```python
from build123d import *

# Parameters (mm, degrees)
F0_R          = 12.5
F1_DEPTH      = 10
F2_DEPTH      = 15
F2_DEPTH_BACK = 5


with BuildPart() as f1:
    # F0 (on Top) → F1 (new body)
    with BuildSketch(Plane.XY):
        with BuildLine():
            ThreePointArc((14.990479, 0.534354), (14.99762, 0.267219), (15, 0))
            ThreePointArc((15, 0), (-1.712048, -14.901976), (-14.609185, 3.401721))
            Line((-14.609185, 3.401721), (-48, -140))
            Line((-48, -140), (-78, -140))
            Line((-78, -140), (-78, -150))
            Line((-78, -150), (50, -150))
            Line((50, -150), (50, -140))
            Line((50, -140), (20, -140))
            Line((20, -140), (14.990479, 0.534354))
        make_face()
        with BuildLine():
            ThreePointArc((-14.609185, 3.401721), (-1.712048, -14.901976), (15, 0))
            ThreePointArc((15, 0), (14.99762, 0.267219), (14.990479, 0.534354))
            ThreePointArc((14.990479, 0.534354), (1.446304, 14.930111), (-14.609185, 3.401721))
        make_face()
        Circle(F0_R, mode=Mode.SUBTRACT)
    extrude(amount=F1_DEPTH)

    # F0 (on Top) → F2 (join, two sides)
    with BuildSketch(Plane.XY) as f2_sk:
        with BuildLine():
            ThreePointArc((-14.609185, 3.401721), (-1.712048, -14.901976), (15, 0))
            ThreePointArc((15, 0), (14.99762, 0.267219), (14.990479, 0.534354))
            ThreePointArc((14.990479, 0.534354), (1.446304, 14.930111), (-14.609185, 3.401721))
        make_face()
        Circle(F0_R, mode=Mode.SUBTRACT)
    extrude(amount=F2_DEPTH)
    extrude(f2_sk.sketch, amount=-F2_DEPTH_BACK)


solid = f1.part
```
CAD build for the part. Positions are in the model's coordinates, mm. A direction names the side the tool comes from. Give positions to 0.01 mm unless a question says otherwise; leave off trailing zeros. Write each loop counter-clockwise with the first axis right and the second up, starting at its lowest first coordinate (ties: lowest second). Pieces come first, ordered by that corner, then holes. Notation, with made-up numbers: M 10,76.25 L 64,76.25 A23 cw 64,91.25 Z; hole C 13.25,-15.5 d5. An arc over 180 degrees is marked long. Return JSON: item names as keys, results as strings. Group by question number.
(1) 3-axis set-ups, long thin cutter, end or side, ignore diameter. For faces 1 (the face through (-63, -140, 5)), 2 (the face through (-3.4, 12.3, 15)), 3 (the face through (35, -140, 5)): which of +Z, -Z, +X, -X, +Y, -Y reach the whole face in a straight line?
(2) Drill centre lines: L1, parallel to Y at x = 0, z = -3.6; L2, parallel to Y at x = 0, z = 7; L3, parallel to Y at x = 39, z = 3.75. Where is each one in solid material? Low to high. Write a range as [from, to].
(3) Band-saw the part on D-D (y = -108). Give the cut face in (x, z), and give its area (3 significant figures).
(4) Band-saw the part on B-B (z = 7.25). Give the cut face in (x, y).
(5) Flat gauge pins, fed straight in: pin 1 Ø1 at (x, y) = (5.5, -70) entering from +Z; pin 2 Ø20 at (x, y) = (0, 0) entering from +Z; pin 3 Ø3 at (x, z) = (40, 4) entering from +Y; pin 4 Ø10 at (x, y) = (-29, -43) entering from -Z. Where does each tip first touch, or does it go through?
(6) Band-saw the part on C-C (z = -2). Give the cut face in (x, y).
(7) Band-saw the part on A-A (x = 0). Give the cut face in (y, z).
Entries:
{
 "1": {"face 1": "+Z, -Z, -X, +Y", "face 2": "+Z, +X, -X, +Y, -Y", "face 3": "+Z, -Z, +X, +Y"},
 "2": {"L1": "y = [-15, -12.5], [12.5, 15]", "L2": "y = [-150, -12.5], [12.5, 15]", "L3": "y = [-150, -140]"},
 "3": {"outline": "M -40.55,0 L 18.86,0 L 18.86,10 L -40.55,10 Z", "area": "594 mm^2"},
 "4": {"outline": "M -78,-150 L 50,-150 L 50,-140 L 20,-140 L 14.99,0.53 A15 ccw -14.61,3.4 L -48,-140 L -78,-140 Z; hole C 0,0 d25"},
 "5": {"pin 1": "stops at z = 10", "pin 2": "passes through", "pin 3": "stops at y = -140", "pin 4": "stops at z = 0"},
 "6": {"outline": "M 14.99,0.53 A15 ccw long 15,0 A15 ccw Z; hole C 0,0 d25"},
 "7": {"outline": "M -150,0 L -15,0 L -15,-5 L -12.5,-5 L -12.5,15 L -15,15 L -15,10 L -150,10 Z; M 12.5,-5 L 15,-5 L 15,15 L 12.5,15 Z"}
}
